Build history of the part. All positions in model axes, mm. Face numbers are marked on the shaded views. A direction names the side the tool comes from. Round coordinates to 2 decimals unless told otherwise and drop trailing zeros. Write each loop counter-clockwise with the first axis right and the second up, starting at its lowest first coordinate (ties: lowest second). Pieces come first, ordered by that corner, then holes.
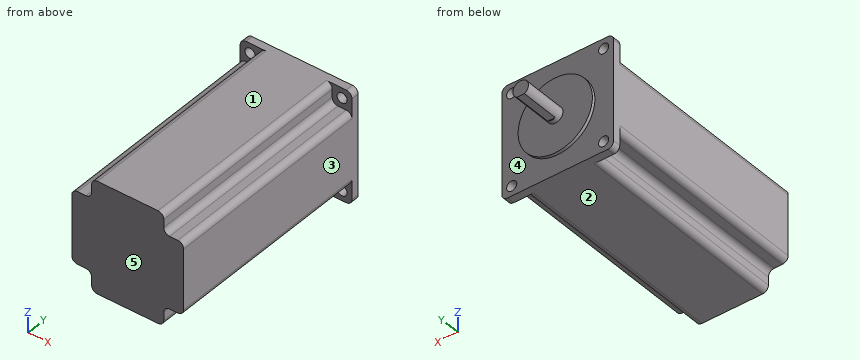
from build123d import *

# Parameters (mm, degrees)
SKETCH1_R           = 2.6
BOSS_EXTRUDE1_DEPTH = 4
SKETCH2_R           = 19.05
BOSS_EXTRUDE2_DEPTH = 1.6
SKETCH3_R           = 4
BOSS_EXTRUDE3_DEPTH = 22.4
CUT_EXTRUDE1_DEPTH  = 20
BOSS_EXTRUDE4_DEPTH = 109


with BuildPart() as part:
    # Sketch1 → Boss-Extrude1 (new body)
    with BuildSketch(Plane(origin=(0, 0, 0), x_dir=(1, 0, 0), z_dir=(0, 1, 0))):
        with BuildLine():
            Line((25.65, -28.65), (-25.65, -28.65))
            ThreePointArc((-25.65, -28.65), (-27.771320344, -27.771320344), (-28.65, -25.65))
            Line((-28.65, -25.65), (-28.65, 25.65))
            ThreePointArc((-28.65, 25.65), (-27.771320344, 27.771320344), (-25.65, 28.65))
            Line((-25.65, 28.65), (25.65, 28.65))
            ThreePointArc((25.65, 28.65), (27.771320344, 27.771320344), (28.65, 25.65))
            Line((28.65, 25.65), (28.65, -25.65))
            ThreePointArc((28.65, -25.65), (27.771320344, -27.771320344), (25.65, -28.65))
        make_face()
        with Locations((-23.57, 23.57)):
            Circle(SKETCH1_R, mode=Mode.SUBTRACT)
        with Locations((23.57, 23.57)):
            Circle(SKETCH1_R, mode=Mode.SUBTRACT)
        with Locations((23.57, -23.57)):
            Circle(SKETCH1_R, mode=Mode.SUBTRACT)
        with Locations((-23.57, -23.57)):
            Circle(SKETCH1_R, mode=Mode.SUBTRACT)
    extrude(amount=-BOSS_EXTRUDE1_DEPTH)

    # Sketch2 → Boss-Extrude2 (add)
    with BuildSketch(Plane(origin=(0, 0, 0), x_dir=(1, 0, 0), z_dir=(0, 1, 0))):
        Circle(SKETCH2_R)
    extrude(amount=BOSS_EXTRUDE2_DEPTH)

    # Sketch3 → Boss-Extrude3 (add)
    with BuildSketch(Plane(origin=(0, 1.6, 0), x_dir=(1, 0, 0), z_dir=(0, 1, 0))):
        Circle(SKETCH3_R)
    extrude(amount=BOSS_EXTRUDE3_DEPTH)

    # Sketch4 → Cut-Extrude1 (cut)
    with BuildSketch(Plane(origin=(0, 24, 0), x_dir=(1, 0, 0), z_dir=(0, 1, 0))):
        with BuildLine():
            Line((-1.936491673, 3.5), (1.936491673, 3.5))
            ThreePointArc((1.936491673, 3.5), (0, 4), (-1.936491673, 3.5))
        make_face()
    extrude(amount=-CUT_EXTRUDE1_DEPTH, mode=Mode.SUBTRACT)

    # Sketch5 → Boss-Extrude4 (add)
    with BuildSketch(Plane.XZ.offset(4)):
        with BuildLine():
            Line((-18.49, 25.65), (-18.49, 21.49))
            ThreePointArc((-18.49, 21.49), (-19.368679656, 19.368679656), (-21.49, 18.49))
            Line((-21.49, 18.49), (-25.65, 18.49))
            ThreePointArc((-25.65, 18.49), (-27.771320344, 17.611320344), (-28.65, 15.49))
            Line((-28.65, 15.49), (-28.65, -15.49))
            ThreePointArc((-28.65, -15.49), (-27.771320344, -17.611320344), (-25.65, -18.49))
            Line((-25.65, -18.49), (-21.49, -18.49))
            ThreePointArc((-21.49, -18.49), (-19.368679656, -19.368679656), (-18.49, -21.49))
            Line((-18.49, -21.49), (-18.49, -25.65))
            ThreePointArc((-18.49, -25.65), (-17.611320344, -27.771320344), (-15.49, -28.65))
            Line((-15.49, -28.65), (15.49, -28.65))
            ThreePointArc((15.49, -28.65), (17.611320344, -27.771320344), (18.49, -25.65))
            Line((18.49, -25.65), (18.49, -21.49))
            ThreePointArc((18.49, -21.49), (19.368679656, -19.368679656), (21.49, -18.49))
            Line((21.49, -18.49), (25.65, -18.49))
            ThreePointArc((25.65, -18.49), (27.771320344, -17.611320344), (28.65, -15.49))
            Line((28.65, -15.49), (28.65, 15.49))
            ThreePointArc((28.65, 15.49), (27.771320344, 17.611320344), (25.65, 18.49))
            Line((25.65, 18.49), (21.49, 18.49))
            ThreePointArc((21.49, 18.49), (19.368679656, 19.368679656), (18.49, 21.49))
            Line((18.49, 21.49), (18.49, 25.65))
            ThreePointArc((18.49, 25.65), (17.611320344, 27.771320344), (15.49, 28.65))
            Line((15.49, 28.65), (-15.49, 28.65))
            ThreePointArc((-15.49, 28.65), (-17.611320344, 27.771320344), (-18.49, 25.65))
        make_face()
    extrude(amount=BOSS_EXTRUDE4_DEPTH)


solid = part.part
1) Mould opens along Z. For the marked faces 1, 2 and 3 say: released by +Z, released by -Z, zero draft, split by the parting line, or undercut.
Results:
face 1: released by +Z
face 2: released by -Z
face 3: zero draft
2) Slice it at B-B (y = -1.5). Write the cut outline in (x, z), plus the area to 3 significant figures.
Results:
outline: (-28.65, -25.65) arc R3 ccw to (-25.65, -28.65) - (25.65, -28.65) arc R3 ccw to (28.65, -25.65) - (28.65, 25.65) arc R3 ccw to (25.65, 28.65) - (-25.65, 28.65) arc R3 ccw to (-28.65, 25.65) - close; hole circle Ø5.2 at (-23.57, -23.57); hole circle Ø5.2 at (-23.57, 23.57); hole circle Ø5.2 at (23.57, -23.57); hole circle Ø5.2 at (23.57, 23.57)
area: 3,190 mm2
3) Slice it at A-A (x = 23.57). Write the cut outline in (y, z), plus the area to 3 significant figures.
Results:
outline: (-113, -18.49) - (-4, -18.49) - (-4, -20.97) - (0, -20.97) - (0, 20.97) - (-4, 20.97) - (-4, 18.49) - (-113, 18.49) - close; (-4, -28.65) - (0, -28.65) - (0, -26.17) - (-4, -26.17) - close; (-4, 26.17) - (0, 26.17) - (0, 28.65) - (-4, 28.65) - close
area: 4,220 mm2
4) Slice it at C-C (z = 23.57). Write the cut outline in (x, y).
Results:
outline: (-28.65, -4) - (-26.17, -4) - (-26.17, 0) - (-28.65, 0) - close; (-20.97, -4) - (-18.49, -4) - (-18.49, -113) - (18.49, -113) - (18.49, -4) - (20.97, -4) - (20.97, 0) - (-20.97, 0) - close; (26.17, -4) - (28.65, -4) - (28.65, 0) - (26.17, 0) - close
5) Wall check: L1, parallel to X at y = -2.2, z = 23.57; L2, parallel to X at y = -1, z = 23. Give the ranges that are in metal, low to high.
Results:
L1: x = -28.65 to -26.17, -20.97 to 20.97, 26.17 to 28.65
L2: x = -28.65 to -26.11, -21.03 to 21.03, 26.11 to 28.65
6) Slice it at D-D (z = 0). Write the cut outline in (x, y), plus the area to 3 significant figures.
Results:
outline: (-28.65, -113) - (28.65, -113) - (28.65, 0) - (19.05, 0) - (19.05, 1.6) - (4, 1.6) - (4, 24) - (-4, 24) - (-4, 1.6) - (-19.05, 1.6) - (-19.05, 0) - (-28.65, 0) - close
area: 6,720 mm2
7) Which spindle directions (+Z, -Z, +X, -X, +Y, -Y) get a long thin tool onto all of the face, cutting with end or side? Do the marked faces 4 and 5. Say none if no direction does.
Results:
face 4: +Y
face 5: +Z, -Z, +X, -X, -Y
8) Pin check, flat tips, straight feed: pin 1 Ø7 at (x, z) = (-23.57, -23.57) entering from -Y; pin 2 Ø2 at (y, z) = (-53.5, -24) entering from +X; pin 3 Ø1 at (x, y) = (17.5, -83) entering from +Z. Stop position of each tip, or through.
Results:
pin 1: stops at y = -4
pin 2: stops at x = 18.49
pin 3: stops at z = 28.24
